The model under review builds one solid part; all positions refer to its coordinate system, in mm. A direction names the side the tool comes from. Give positions to 0.01 mm unless a question says otherwise; leave off trailing zeros. Order: outer loops, then holes, each group sorted by start corner. A loop starts at its lowest first (then second) coordinate and runs counter-clockwise, first axis right, second up. Notation, with made-up numbers: (55, 55.25) - (95, 55.25) arc R17 ccw to (95, 61.25) - close; hole circle Ø5 at (-1.75, -15). An arc over 180 degrees is marked (long way). Use CSV: the item, a comma, the result in double quotes. Start each with the question number.
1. Take a section at D-D, the plane z = 40. State the section outline as (x, y) points (3 decimals), then the cut area to 3 significant figures.
2. Take a section at A-A, the plane z = 30. State the section outline as (x, y) points (3 decimals), then the cut area to 3 significant figures.
3. Draft analysis for pull direction Z (two halves, no side actions). For faces 1 (the cylindrical face through (2.89, 1.57, 1.86)), 2 (the flat face through (-51, 2, 0)), 3 (the flat face through (-35.16, 1.57, 32.79)), state which applies: released by +Z, released by -Z, zero draft, split by the parting line, or undercut.
4. Take a section at B-B, the plane x = -12.5. State the section outline as (y, z) points (3 decimals), then the cut area to 3 significant figures.
5. To check wall thickness, follow line 1 (Z direction, x = -11, y = 1.6); line 2 (Z direction, x = -16, y = 2.5); line 3 (Z direction, x = -63.5, y = 0.2). State the ranges of each line that lie inside material, in increasing order. Write a range as [from, to].
6. Take a section at C-C, the plane y = 2.5. State the section outline as (x, z) points (1 decimal).
7. For pin 1 (5 mm diameter, centred on x = -43.53, z = 13.29, fed in from -Y); pin 2 (3.5 mm diameter, centred on x = -81.63, z = 13.29, fed in from +Y); pin 3 (1 mm diameter, centred on y = 0.5, z = 7.5, fed in from +X); pin 4 (1 mm diameter, centred on x = -22.5, y = 0.5, fed in from +Z), all flat-tipped, find the tip position at first contact; note any pin that passes through.
8. Machinability: for faces 4 (the cylindrical face through (-12.376, 1.565, 24.614)), 5 (the flat face through (-93.51, 1.57, 30.26)), 6 (the flat face through (-71.908, 1.565, 29.184)), which of the approach directions +Z, -Z, +X, -X, +Y, -Y give a long, thin tool a straight path to every point of the face, cutting with its end or side? Answer none if there is none.
Autodesk Inventor part; units mm, degrees
ref_plane "YZ Plane" through (0, 0, 0) normal (1, 0, 0) x (0, 1, 0)
ref_plane "XZ Plane" through (0, 0, 0) normal (0, 1, 0) x (-1, 0, 0)
ref_plane "XY Plane" through (0, 0, 0) normal (0, 0, 1) x (1, 0, 0)
sketch "Sketch1" plane through (0, 0, 0) normal (0, 1, 0) x (-1, 0, 0)
  line L0 (1.8157, 35.2839) -> (-2.8584, 20.966)
  arc A0 (-2.8584, 20.966) -> (-1.9975, 17.6511) centre (0.1598, 19.9807) ccw
  line L1 (-1.9975, 17.6511) -> (-0.6941, 16.4441)
  arc A1 (-0.3495, 7.4705) -> (-0.6941, 16.4441) centre (-5.0086, 11.785) ccw
  line L2 (-0.3495, 7.4705) -> (-2.3296, 5.3323)
  arc A2 (-2.3296, 5.3323) -> (0, 0) centre (0, 3.175) ccw
  line L3 (0, 0) -> (102.7651, 0)
  arc A3 (102.7651, 0) -> (111.9831, 2.3787) centre (102.7651, 19.05) ccw
  arc A4 (111.9831, 2.3787) -> (111.0681, 4.7241) centre (111.3685, 3.4901) ccw
  arc A5 (92.5709, 28.4903) -> (111.0681, 4.7241) centre (107.1622, 20.7654) ccw
  line L4 (92.5709, 28.4903) -> (94.4719, 32.0811)
  arc A6 (94.4719, 32.0811) -> (92.6849, 34.3642) centre (93.0689, 32.8239) ccw
  line L5 (92.6849, 34.3642) -> (50.542, 23.8568)
  line L6 (50.542, 23.8568) -> (19.3436, 41.9732)
  arc A7 (19.3436, 41.9732) -> (1.8157, 35.2839) centre (13.285, 31.5396) ccw
  circle A8 centre (43.5324, 13.2882) radius 2.2479
  circle A9 centre (81.6324, 13.2882) radius 2.2479
  circle A10 centre (13.285, 31.5396) radius 6.985
  point P0 (0, 0)
  point P1 (19.3436, 41.9732)
  point P2 (-1.9975, 17.6511)
  point P3 (-0.6941, 16.4441)
  point P4 (0, 0)
  point P5 (111.9831, 2.3787)
  point P6 (111.0681, 4.7241)
extrude "Plate1" add sketch "Sketch1" along normal blind 3.175
equation "\"d0\" = Thickness"
equation "\"BendRadius\" = Thickness"
equation "\"BendReliefWidth\" = Thickness"
equation "\"BendReliefDepth\" = 0.5 * Thickness"
equation "\"CornerReliefSize\" = 4 * Thickness"
equation "\"MinimumRemnant\" = 2 * Thickness"
equation "\"TransitionRadius\" = BendRadius"
equation "\"JacobiRadiusSize\" = BendRadius"
equation "\"GapSize\" = Thickness"
properties part number "hook-bottom-plate" material "Aluminum 6061"
Determined:
1,outline,"(-22.742, 0) - (-4.683, 0) - (-4.683, 3.175) - (-22.742, 3.175) - close"
1,area,"57.3 mm²"
2,outline,"(-93.37, 0) - (-75.181, 0) - (-75.181, 3.175) - (-93.37, 3.175) - close; (-39.963, 0) - (-20.098, 0) - (-20.098, 3.175) - (-39.963, 3.175) - close; (-6.472, 0) - (-0.091, 0) - (-0.091, 3.175) - (-6.472, 3.175) - close"
2,area,"141 mm²"
3,face 1,"undercut"
3,face 2,"released by -Z"
3,face 3,"released by +Z"
4,outline,"(0, 0) - (3.175, 0) - (3.175, 24.599) - (0, 24.599) - close; (0, 38.48) - (3.175, 38.48) - (3.175, 43.579) - (0, 43.579) - close"
4,area,"94.3 mm²"
5,line 1,"z = [0, 24.94], [38.14, 43.39]"
5,line 2,"z = [0, 25.1], [37.98, 43.3]"
5,line 3,"z = [0, 27.09]"
6,outline,"(-112, 2.4) arc R19.1 ccw to (-102.8, 0) - (0, 0) arc R3.2 ccw to (2.3, 5.3) - (0.3, 7.5) arc R6.3 cw to (0.7, 16.4) - (2, 17.7) arc R3.2 ccw to (2.9, 21) - (-1.8, 35.3) arc R12.1 ccw to (-19.3, 42) - (-50.5, 23.9) - (-92.7, 34.4) arc R1.6 ccw to (-94.5, 32.1) - (-92.6, 28.5) arc R16.5 cw to (-111.1, 4.7) arc R1.3 ccw to start; hole circle Ø4.5 at (-81.6, 13.3); hole circle Ø4.5 at (-43.5, 13.3); hole circle Ø14 at (-13.3, 31.5)"
7,pin 1,"stops at y = 0"
7,pin 2,"passes through"
7,pin 3,"stops at x = 0.79"
7,pin 4,"stops at z = 40.43"
8,face 4,"+Y, -Y"
8,face 5,"-X, +Y, -Y"
8,face 6,"+Z, +Y, -Y"
